Study the drawing (mm; zero at the part's minimum x, y, z) and answer. Give positions to 0.01 mm unless a question says otherwise; leave off trailing zeros. Order: outer loops, then holes, each group sorted by start corner. A loop starts at its lowest first (then second) coordinate and runs counter-clockwise, first axis right, second up.
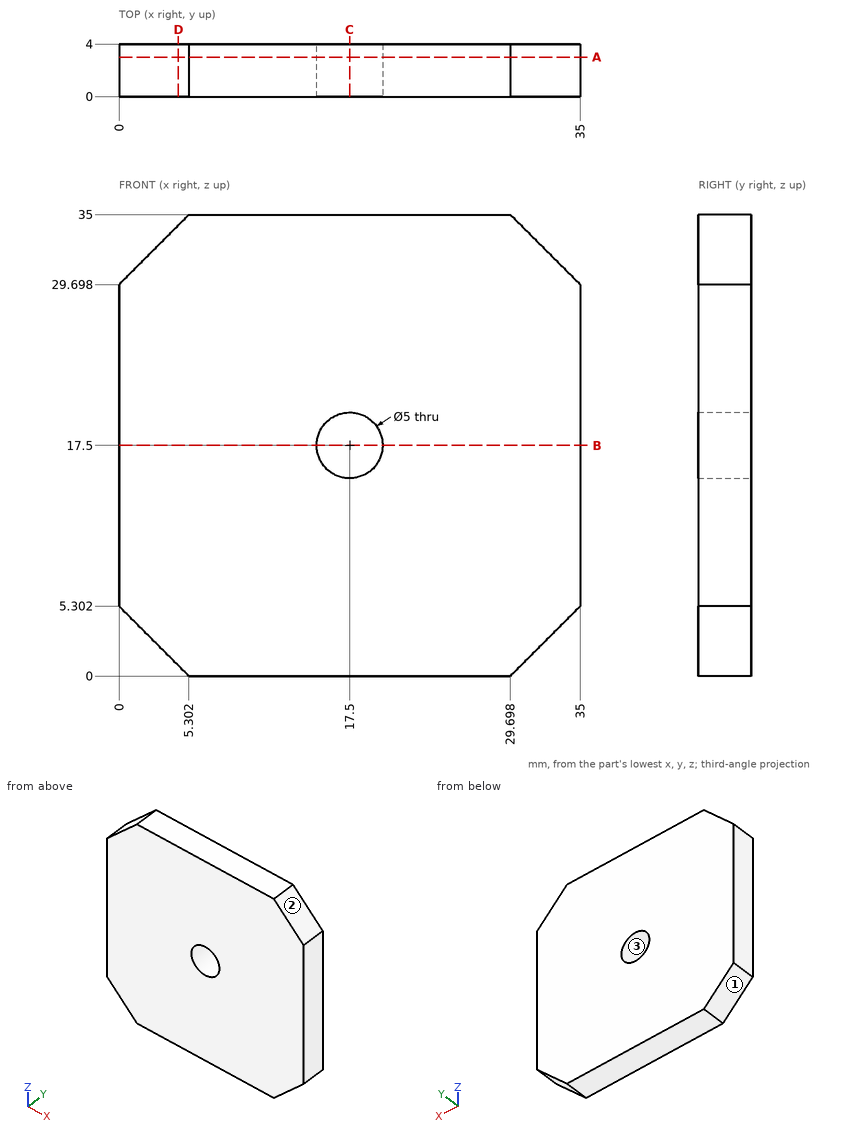
1) Find section A-A (y = 3). Write down the section's boundary in (x, z).
Geometry says:
outline: (0, 5.3) - (5.3, 0) - (29.7, 0) - (35, 5.3) - (35, 29.7) - (29.7, 35) - (5.3, 35) - (0, 29.7) - close; hole circle Ø5 at (17.5, 17.5)
2) Find section D-D (x = 4.5). Write down the section's boundary in (y, z), then the cut area to 3 significant figures.
Geometry says:
outline: (0, 0.8) - (4, 0.8) - (4, 34.2) - (0, 34.2) - close
area: 134 mm2
3) Find section C-C (x = 17.5). Write down the section's boundary in (y, z).
Geometry says:
outline: (0, 0) - (4, 0) - (4, 15) - (0, 15) - close; (0, 20) - (4, 20) - (4, 35) - (0, 35) - close
4) For a pull along Z with two mould halves and no side action, classify the marked faces 1, 2 and 3 as +Z half, -Z half, draft (parallel to the pull), parting line (faces both ways), or undercut.
Geometry says:
face 1: -Z half
face 2: +Z half
face 3: undercut
5) Straight lines are drawn through the part: probe 1 along X at (y, z) = (1.9, 17.5); probe 2 along X at (y, z) = (0.25, 16). For each, find the intervals that lie inside material, in ascending order.
Geometry says:
probe 1: x = 0 to 15, 20 to 35
probe 2: x = 0 to 15.5, 19.5 to 35
6) Find section B-B (z = 17.5). Write down the section's boundary in (x, y), then the cut area to 3 significant figures.
Geometry says:
outline: (0, 0) - (15, 0) - (15, 4) - (0, 4) - close; (20, 0) - (35, 0) - (35, 4) - (20, 4) - close
area: 120 mm2
